```python
from build123d import *

# Parameters (mm, degrees)
F1_DEPTH = 25.4
F3_DEPTH = 2.54
F4_DEPTH = 2.54
F6_DEPTH = 25.4


with BuildPart() as f1:
    # F0 (on Top) → F1 (new body)
    with BuildSketch(Plane.XY):
        Polygon((35.4939039202, 3.9029268082), (12.342310436, -26.2274350854), (15.2102268336, -26.2274350854), (38.3618203178, 3.9029268082), (17.5462131575, 31.9668278098), (11.970603764, 26.2053646147), (14.0355655072, 24.2070145946), (17.4720109704, 27.7580083355), (17.4720109704, 15.9834139049), (-16.084820535, 15.9834139049), (-49.6416520405, 15.9834139049), (-49.6416520405, 27.7580083355), (-46.2052065773, 24.2070145946), (-44.1402448341, 26.2053646147), (-49.7158542275, 31.9668278098), (-70.5314613879, 3.9029268082), (-47.3798679037, -26.2274350854), (-44.5119515061, -26.2274350854), (-67.6635449903, 3.9029268082), (-62.1494763114, 11.3370735198), (-16.084820535, 11.3370735198), (29.9798352413, 11.3370735198), align=None)
        Polygon((-51.9630546496, 25.6478060037), (-51.9630546496, 15.7975610346), (-59.2113519833, 15.7975610346), align=None, mode=Mode.SUBTRACT)
        Polygon((19.7934135795, 15.7975610346), (19.7934135795, 25.6478060037), (27.0417109132, 15.7975610346), align=None, mode=Mode.SUBTRACT)
    extrude(amount=F1_DEPTH)

    # F2 (on face) → F3 (cut)
    with BuildSketch(Plane(origin=(-42.4623607514, -32.6272654131, 0), x_dir=(0.6092872739, -0.7929495683, 0), z_dir=(-0.7929495683, -0.6092872739, 0))):
        with BuildLine():
            Line((-8.0709172227, 25.4), (-46.0687459593, 25.4))
            add(Edge.make_bspline(
                [(-46.0687459593, 25.4), (-40.915928781, 17.5322014838), (-30.6555183473, 9.8364153651), (-15.6398303807, 8.4253717214), (-8.0709172227, 0)],
                knots=[0, 0, 0, 0, 0.4807876379, 1, 1, 1, 1], degree=3))
            Line((-8.0709172227, 0), (-8.0709172227, 25.4))
        make_face()
    extrude(amount=-F3_DEPTH, mode=Mode.SUBTRACT)

    # F0 (on Top) → F4 (join)
    with BuildSketch(Plane.XY):
        Polygon((-44.5119515061, -26.2274350854), (-16.084820535, -26.2274350854), (12.342310436, -26.2274350854), (35.4939039202, 3.9029268082), (29.9798352413, 11.3370735198), (-16.084820535, 11.3370735198), (-62.1494763114, 11.3370735198), (-67.6635449903, 3.9029268082), align=None)
        Polygon((35.4939039202, 3.9029268082), (12.342310436, -26.2274350854), (15.2102268336, -26.2274350854), (38.3618203178, 3.9029268082), (17.5462131575, 31.9668278098), (11.970603764, 26.2053646147), (14.0355655072, 24.2070145946), (17.4720109704, 27.7580083355), (17.4720109704, 15.9834139049), (-16.084820535, 15.9834139049), (-49.6416520405, 15.9834139049), (-49.6416520405, 27.7580083355), (-46.2052065773, 24.2070145946), (-44.1402448341, 26.2053646147), (-49.7158542275, 31.9668278098), (-70.5314613879, 3.9029268082), (-47.3798679037, -26.2274350854), (-44.5119515061, -26.2274350854), (-67.6635449903, 3.9029268082), (-62.1494763114, 11.3370735198), (-16.084820535, 11.3370735198), (29.9798352413, 11.3370735198), align=None)
        Polygon((-51.9630546496, 25.6478060037), (-51.9630546496, 15.7975610346), (-59.2113519833, 15.7975610346), align=None, mode=Mode.SUBTRACT)
        Polygon((19.7934135795, 15.7975610346), (19.7934135795, 25.6478060037), (27.0417109132, 15.7975610346), align=None, mode=Mode.SUBTRACT)
        Polygon((-59.2113519833, 15.7975610346), (-51.9630546496, 15.7975610346), (-51.9630546496, 25.6478060037), align=None)
    extrude(amount=-F4_DEPTH)

    # F5 (on face) → F6 (join)
    with BuildSketch(Plane(origin=(0, 0, -2.54), x_dir=(1, 0, 0), z_dir=(0, 0, -1))):
        Polygon((-49.6416520405, -15.9834139049), (-33.3581715822, -15.9834139049), (-33.3581715822, -11.3370744511), (-62.1654912829, -11.3370744511), (-58.0767057836, -15.9834139049), align=None)
    extrude(amount=F6_DEPTH)


solid = f1.part
```
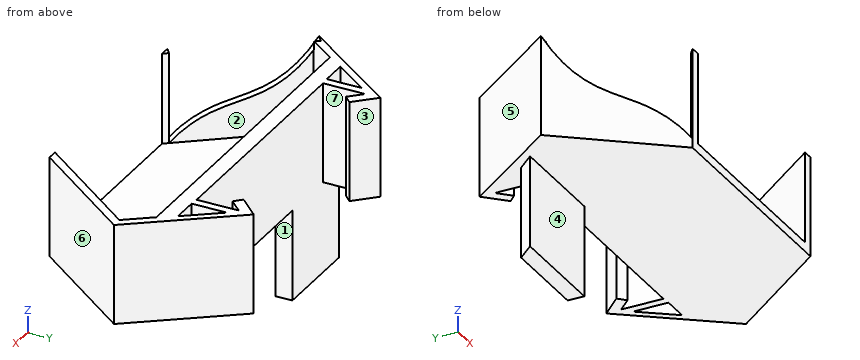
Build history of the part. All positions in model axes, mm. Face numbers are marked on the shaded views. A direction names the side the tool comes from. Round coordinates to 2 decimals unless told otherwise and drop trailing zeros. Write each loop counter-clockwise with the first axis right and the second up, starting at its lowest first coordinate (ties: lowest second). Pieces come first, ordered by that corner, then holes. Notation, with made-up numbers: (60, 7.5) - (98, 7.5) arc R29 ccw to (98, 36.5) - close; hole circle Ø11 at (-22, -32). An arc over 180 degrees is marked (long way). Answer as CSV lines item,"result".
Q1. Cut at A-A (y = 17.5). Write the cut outline in (x, z), and give its area (3 significant figures).
Report:
outline,"(-60.45, -2.54) - (-49.64, -2.54) - (-49.64, 25.4) - (-51.96, 25.4) - (-51.96, 0) - (-57.96, 0) - (-57.96, 25.4) - (-60.45, 25.4) - close; (17.47, -2.54) - (19.79, -2.54) - (19.79, 25.4) - (17.47, 25.4) - close; (25.79, -2.54) - (28.28, -2.54) - (28.28, 25.4) - (25.79, 25.4) - close"
area,"284 mm^2"
Q2. Cut at C-C (z = 3.5). State how many separate pieces and enclosed holes the cut face has, and give its area (3 significant figures).
Report:
separate pieces,"2"
enclosed holes,"2"
area,"803 mm^2"
Q3. Pull direction X, two halves, no side cores. Call the marked faces 5, 6 and 7: +X half, -X half, draft (parallel to the pull), parting line (faces both ways), or undercut.
Report:
face 5,"-X half"
face 6,"+X half"
face 7,"undercut"
Q4. Drill centre lines: probe 1 along Z at (x, y) = (-50, 9.5); probe 2 along Z at (x, y) = (-28.5, 14); probe 3 along Y at (x, z) = (-48, 14). Where is each one in solid material? Low to high. Write a range as [from, to].
Report:
probe 1,"z = [-2.54, 0]"
probe 2,"z = [-2.54, 25.4]"
probe 3,"y = [11.34, 15.98], [26.06, 30.19]"
Q5. Cut at B-B (x = 9). Write the cut outline in (y, z).
Report:
outline,"(-26.23, -2.54) - (15.98, -2.54) - (15.98, 25.4) - (11.34, 25.4) - (11.34, 0) - (-26.23, 0) - close"
Q6. Tool access for the marked faces 1, 2, 3 and 4: list every direction of +Z, -Z, +X, -X, +Y, -Y with a clear straight run to the whole face (end or side of a thin tool).
Report:
face 1,"-Z, +X, +Y, -Y"
face 2,"+Z"
face 3,"+Z, -Z, +Y"
face 4,"-Z, +X, -X, -Y"
Q7. Cut at D-D (x = 24). Write the cut outline in (y, z), and give its area (3 significant figures).
Report:
outline,"(-14.79, -2.54) - (15.8, -2.54) - (15.8, 25.4) - (11.34, 25.4) - (11.34, 0) - (-11.06, 0) - (-11.06, 25.4) - (-14.79, 25.4) - close; (19.93, -2.54) - (23.27, -2.54) - (23.27, 25.4) - (19.93, 25.4) - close"
area,"379 mm^2"
Q8. Drop flat-ended pins along their axis: pin 1 (2 mm diameter, centred on x = -47, y = 7.5, fed in from +Z); pin 2 (5 mm diameter, centred on y = 14.5, z = -12, fed in from +X); pin 3 (8 mm diameter, centred on x = -55.5, z = 9.5, fed in from +Y). Give the stop position or say it passes through.
Report:
pin 1,"stops at z = 0"
pin 2,"stops at x = -33.36"
pin 3,"stops at y = 29.56"
